For this review, take the finished solid that the model builds, in its own axes (mm). Face numbers are marked on the shaded views. A direction names the side the tool comes from. Coordinates: 2 decimals unless noted, no trailing zeros. Write each loop counter-clockwise with the first axis right and the second up, starting at its lowest first coordinate (ties: lowest second). Pieces come first, ordered by that corner, then holes. Notation, with made-up numbers: (-36.75, 44) - (8.25, 44) arc R20 ccw to (8.25, 58) - close; hole circle Ø6 at (-3, 48.25). An arc over 180 degrees is marked (long way). Use one line per item in the form item = value. Start each with the question number.
1) We need section A-A (z = 69). Give the boundary of the cut face in (x, y).
2) We need section B-B (x = 66). Give the boundary of the cut face in (y, z).
3) Tool access review of the marked faces 4, 5 and 6: name each direction out of +Z, -Z, +X, -X, +Y, -Y from which nothing blocks a thin tool from reaching the whole face with its end or side.
4) We need section C-C (y = -43). Give the boundary of the cut face in (x, z), plus the area to 3 significant figures.
5) We need section D-D (y = -11.5). Give the boundary of the cut face in (x, z), plus the area to 3 significant figures.
6) Mouldability with a two-part tool opening along X and no side actions: class the marked faces 1, 2 and 3 as pulls with the +X half, pulls with the -X half, needs draft (parallel to the pull), parting line crosses it, or undercut.
7) Insertion check: P1, Ø3, axis at x = -14.5, z = 13.5, coming from the +Y side; P2, Ø8, axis at x = 0.5, z = 48.5, coming from the -Y side; P3, Ø10, axis at x = 33.5, z = 41.5, coming from the +Y side. Each pin has a flat end and moves straight along its axis. Give the tip position at first contact, or say it passes through.
8) For L1, parallel to X at y = -17, z = 64; L2, parallel to X at y = -103, z = 62; L3, parallel to Z at x = 73, y = -84, list the stretches that pass through material, from the lowest coordinate up. Write a range as from..to.
```python
from build123d import *

# Parameters (mm, degrees)
F0_W        = 127
F0_H        = 120.65
F1_DEPTH    = 76.2
F2_T1_DEPTH = 687.8168150118
F3_W        = 76.2
F3_H        = 31.75
F4_DEPTH    = 76.2
F5_R        = 9.9779768357
F6_DEPTH    = 215.9


# Not quite as in the source:
# - a fillet or chamfer that OpenCascade refuses, or shapes differently, is made with other operations: its cross-section is extruded or revolved along the edge and cut away or added


with BuildPart() as f1:
    # F0 (on Top) → F1 (new body)
    with BuildSketch(Plane.XY):
        with Locations((25.4407467544, -4.8593845844)):
            Rectangle(F0_W, F0_H)
    extrude(amount=F1_DEPTH)

    # F2: fillet of radius 120.65 on 1 edges, made by hand

    # F2_s2 → F2_t1 (cut)
    with BuildSketch(Plane.YZ.offset(-318.4676607515)):
        with BuildLine():
            ThreePointArc((55.4656154156, 0), (11.1016993136, 55.3480836489), (-56.6977475868, 76.2))
            Line((-56.6977475868, 76.2), (55.4656154156, 76.2))
            Line((55.4656154156, 76.2), (55.4656154156, 0))
        make_face()
    extrude(amount=F2_T1_DEPTH, mode=Mode.SUBTRACT)

    # F3 (on face) → F4 (join)
    with BuildSketch(Plane.XZ.offset(65.1843845844)):
        with Locations((50.8407467544, 60.325)):
            Rectangle(F3_W, F3_H)
    extrude(amount=F4_DEPTH)

    # F5 (on face) → F6 (cut)
    with BuildSketch(Plane.XZ.offset(141.3843845844)):
        with Locations((50.7810004056, 63.9038160443)):
            Circle(F5_R)
    extrude(amount=-F6_DEPTH, mode=Mode.SUBTRACT)


solid = f1.part
```
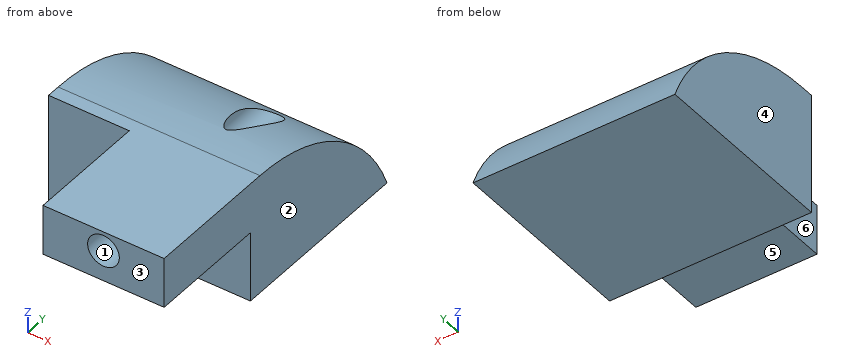
Determined:
q1.outline = (-38.06, -65.18) - (12.74, -65.18) - (12.74, -141.38) - (42.2, -141.38) - (42.2, -15.64) - (-38.06, -15.64) - close; (59.36, -141.38) - (88.94, -141.38) - (88.94, -15.64) - (59.36, -15.64) - close
q2.outline = (-141.38, 44.45) - (-65.18, 44.45) - (-65.18, 0) - (55.47, 0) arc R120.65 ccw to (-56.7, 76.2) - (-141.38, 76.2) - close
q3.face_4 = +Z, -Z, -X, +Y, -Y
q3.face_5 = -Z, +X, -X, -Y
q3.face_6 = +Z, -Z, -X, -Y
q4.outline = (-38.06, 0) - (88.94, 0) - (88.94, 75.42) - (-38.06, 75.42) - close; hole circle Ø19.96 at (50.78, 63.9)
q4.area = 9,270 mm²
q5.outline = (-38.06, 0) - (88.94, 0) - (88.94, 67.41) - (60.12, 67.41) arc R9.98 cw (long way) to (41.44, 67.41) - (-38.06, 67.41) - close
q5.area = 8,340 mm²
q6.face_1 = undercut
q6.face_2 = pulls with the +X half
q6.face_3 = needs draft
q7.P1 = 49.93
q7.P2 = -65.18
q7.P3 = 32.76
q8.L1 = -38.06..40.8, 60.76..88.94
q8.L2 = 12.74..40.99, 60.58..88.94
q8.L3 = 44.45..76.2
